Build history of the part. All positions in model axes, mm. A direction names the side the tool comes from. Give positions to 0.01 mm unless a question says otherwise; leave off trailing zeros. Order: outer loops, then holes, each group sorted by start corner. A loop starts at its lowest first (then second) coordinate and runs counter-clockwise, first axis right, second up. Notation, with made-up numbers: (57, 30) - (82, 30) arc R12 cw to (82, 46) - close; hole circle Ø1 at (50, -33.5). An arc over 180 degrees is marked (long way). Write each question's results on one line, items separated by ' | '. Start each with the question number.
1) Drop flat-ended pins along their axis: pin 1 Ø1.2 at (x, z) = (12, -1.5) entering from -Y; pin 2 Ø1.1 at (y, z) = (-14, 1) entering from +X; pin 3 Ø4 at (x, z) = (-12.5, 2) entering from +Y; pin 4 Ø2.5 at (x, z) = (-3, 1) entering from -Y. Give the stop position or say it passes through.
2) Cut at A-A on y = -17. List the corners of the cut face in (x, z).
3) Cut at B-B on x = 3.5. List the corners of the cut face in (y, z).
4) Drill centre lines: line 1 along X through (y, z) = (-14.25, 3); line 2 along Y through (x, z) = (4, -2.25); line 3 along Y through (x, z) = (-5.25, -2). Where is each one in solid material? Low to high. Write a range as from..to.
5) Cut at C-C on y = -9.75. List the corners of the cut face in (x, z).
6) Tool access for faces 1 (the face through (-10, -13.081, 0)), 2 (the face through (-12.86, -4.51, 0.12)), 3 (the face through (-6, -18.847, 0)), 4 (the face through (-10, -13.868, 0)), 5 (the face through (-9, -16.434, 3)): list every direction of +Z, -Z, +X, -X, +Y, -Y with a clear straight run to the whole face (end or side of a thin tool).
7) Two-plate mould, pull along Y, no slides. Class faces 6 (the face through (-12.86, -4.51, -0.74)), 7 (the face through (-3, -18.847, 0)), 8 (the face through (0, -8, 4.083)), 9 (the face through (-12.86, -4.51, 0.98)): +Y half, -Y half, draft (parallel to the pull), parting line (faces both ways), or undercut.
from build123d import *

# Parameters (mm, degrees)
F0_W      = 19.4564
F0_H      = 8.1661
F1_DEPTH  = 16.4338
F3_DEPTH  = 8.1661
F5_DEPTH  = 2.413
F6_R      = 0.635
F7_DEPTH  = 3.5941
F9_R      = 1.0668
F10_DEPTH = 0.7874
F11_R     = 0.40005
F12_DEPTH = 6.35


# Not quite as in the source:
# - a pattern or mirror of a feature is missing from the dataset's text; its kind, count and spacing are read off the source's solid


with BuildPart() as f1:
    # F0 (on Front) → F1 (new body)
    with BuildSketch(Plane.XZ):
        Rectangle(F0_W, F0_H)
    extrude(amount=F1_DEPTH)

    # F2 (on face) → F3 (cut, through all)
    with BuildSketch(Plane(origin=(0, 0, -4.08305), x_dir=(1, 0, 0), z_dir=(0, 0, -1))):
        Polygon((3.9751, 16.4338), (9.7282, 14.8336), (9.7282, 16.4338), align=None)
    extrude(amount=-F3_DEPTH, mode=Mode.SUBTRACT)

    # F4 (on face) → F5 (join)
    with BuildSketch(Plane.XZ.offset(16.4338)):
        with BuildLine():
            ThreePointArc((-2.0754022956, -1.9819683724), (-3.3782, 0), (-2.0754022956, 1.9819683724))
            ThreePointArc((-2.0754022956, 1.9819683724), (-2.1263891254, 2.071139592), (-2.1796029577, 2.159))
            ThreePointArc((-2.1796029577, 2.159), (-3.6632327094, 3.5697760652), (-5.6451500171, 4.08305))
            ThreePointArc((-5.6451500171, 4.08305), (-8.532302349, 2.8871523369), (-9.7282, 0))
            ThreePointArc((-9.7282, 0), (-8.5323023429, -2.8871523429), (-5.64515, -4.08305))
            ThreePointArc((-5.64515, -4.08305), (-3.663232702, -3.5697760611), (-2.1796029577, -2.159))
            ThreePointArc((-2.1796029577, -2.159), (-2.1263891254, -2.071139592), (-2.0754022956, -1.9819683724))
        make_face()
        with BuildLine():
            ThreePointArc((-2.0754022956, -1.9819683724), (-1.6925081197, -1.023679378), (-1.5621, 0))
            ThreePointArc((-1.5621, 0), (-1.6925081197, 1.023679378), (-2.0754022956, 1.9819683724))
            ThreePointArc((-2.0754022956, 1.9819683724), (-3.3782, 0), (-2.0754022956, -1.9819683724))
        make_face()
        with BuildLine():
            ThreePointArc((-2.0754022956, 1.9819683724), (-1.6925081197, 1.023679378), (-1.5621, 0))
            ThreePointArc((-1.5621, 0), (-1.6925081197, -1.023679378), (-2.0754022956, -1.9819683724))
            ThreePointArc((-2.0754022956, -1.9819683724), (-1.656356313, -2.1142789215), (-1.2192, -2.159))
            ThreePointArc((-1.2192, -2.159), (0.3074435406, -1.5266435406), (0.9398, 0))
            ThreePointArc((0.9398, 0), (0.3074435406, 1.5266435406), (-1.2192, 2.159))
            ThreePointArc((-1.2192, 2.159), (-1.656356313, 2.1142789215), (-2.0754022956, 1.9819683724))
        make_face()
    extrude(amount=F5_DEPTH)

    # F6 (on face) → F7 (join)
    with BuildSketch(Plane.XZ.offset(18.8468)):
        Polygon((-5.4271647327, 1.6557624907), (-5.64515, 1.79705), (-5.8631352673, 1.6557624907), (-6.110260765, 1.7358170061), (-6.2842504662, 1.5429250133), (-6.543675, 1.5562909519), (-6.6618120245, 1.324939746), (-6.9158562411, 1.2707062411), (-6.970089746, 1.0166620245), (-7.2014409519, 0.898525), (-7.1880750133, 0.6391004662), (-7.3809670061, 0.465110765), (-7.3009124907, 0.2179852673), (-7.4422, 0), (-7.3009124907, -0.2179852673), (-7.3809670061, -0.465110765), (-7.1880750133, -0.6391004662), (-7.2014409519, -0.898525), (-6.970089746, -1.0166620245), (-6.9158562411, -1.2707062411), (-6.6618120245, -1.324939746), (-6.543675, -1.5562909519), (-6.2842504662, -1.5429250133), (-6.110260765, -1.7358170061), (-5.8631352673, -1.6557624907), (-5.64515, -1.79705), (-5.4271647327, -1.6557624907), (-5.180039235, -1.7358170061), (-5.0060495338, -1.5429250133), (-4.746625, -1.5562909519), (-4.6284879755, -1.324939746), (-4.3744437589, -1.2707062411), (-4.320210254, -1.0166620245), (-4.0888590481, -0.898525), (-4.1022249867, -0.6391004662), (-3.9093329939, -0.465110765), (-3.9893875093, -0.2179852673), (-3.8481, 0), (-3.9893875093, 0.2179852673), (-3.9093329939, 0.465110765), (-4.1022249867, 0.6391004662), (-4.0888590481, 0.898525), (-4.320210254, 1.0166620245), (-4.3744437589, 1.2707062411), (-4.6284879755, 1.324939746), (-4.746625, 1.5562909519), (-5.0060495338, 1.5429250133), (-5.180039235, 1.7358170061), align=None)
        with Locations((-5.64515, 0)):
            Circle(F6_R, mode=Mode.SUBTRACT)
    extrude(amount=F7_DEPTH)

    # F9 (on offset) → F10 (join)
    with BuildSketch(Plane.XZ.offset(13.081)):
        with BuildLine():
            Line((12.0777, 4.08305), (9.7282, 4.08305))
            Line((9.7282, 4.08305), (9.7282, -4.08305))
            Line((9.7282, -4.08305), (12.0777, -4.08305))
            ThreePointArc((12.0777, -4.08305), (13.5763, 0), (12.0777, 4.08305))
        make_face()
        with Locations((11.557, 0)):
            Circle(F9_R, mode=Mode.SUBTRACT)
    f10 = extrude(amount=F10_DEPTH)

    # F10_copies: F10 across plane
    add(f10.mirror(Plane(origin=(0, 0, 0), x_dir=(0, 0, -1), z_dir=(-1, 0, 0))))

    # F11 (on face) → F12 (join)
    with BuildSketch(Plane(origin=(-9.7282, 0, 0), x_dir=(0, -1, 0), z_dir=(-1, 0, 0))):
        with Locations((4.1275, 0.8636)):
            Circle(F11_R)
        with Locations((4.1275, 0)):
            Circle(F11_R)
        with Locations((4.1275, -0.8636)):
            Circle(F11_R)
    extrude(amount=F12_DEPTH)


solid = f1.part
Results:
1) pin 1: y = -13.87 | pin 2: x = 13.56 | pin 3: y = -3.73 | pin 4: y = -22.44
2) outline: (-2.08, -1.98) arc R2.16 ccw (long way) to (-2.08, 1.98) arc R4.08 ccw (long way) to start
3) outline: (-16.43, -4.08) - (0, -4.08) - (0, 4.08) - (-16.43, 4.08) - close
4) line 1: -9.73..9.73 | line 2: -16.43..0 | line 3: -18.85..0
5) outline: (-9.73, -4.08) - (9.73, -4.08) - (9.73, 4.08) - (-9.73, 4.08) - close
6) face 1: +Z, -Z, -X | face 2: -X | face 3: -Y | face 4: +Z, -Z, -X, -Y | face 5: +Z, -X, -Y
7) face 6: undercut | face 7: -Y half | face 8: draft | face 9: undercut
